Job drawing, mm, ordinate dimensions from the low corner. One solid piece. Give positions to 0.01 mm unless a question says otherwise; leave off trailing zeros. Order: outer loops, then holes, each group sorted by start corner. A loop starts at its lowest first (then second) coordinate and runs counter-clockwise, first axis right, second up. Notation, with made-up numbers: (28.25, 14) -> (77.25, 14) arc R22 ccw to (77.25, 42) -> close; hole circle Ø4 at (47, 51). An arc over 180 degrees is marked (long way). Write item = value, one per line. Start each with the question number.
(1) Two-plate mould, pull along X, no slides. Class the marked faces 1, 2 and 3: pulls with the +X half, pulls with the -X half, needs draft (parallel to the pull), parting line crosses it, or undercut.
(2) Saw through at A-A, the plane y = 12.5. List the corners of the cut face in (x, z).
(3) Saw through at C-C, the plane x = 8.25. State how many separate pieces and enclosed holes the cut face has, then the cut area to 3 significant figures.
(4) Probe line 1 along Y through (x, z) = (11.5, 14.5); line 2 along Y through (x, z) = (18.75, 17) (1 decimal); line 3 along X through (y, z) = (8, 10.25). List the from-to ranges inside material, lowest first. Write a range as from..to.
(5) Flat gauge pin, fed straight in: pin 1 (2.5 mm diameter, centred on y = 2.46, z = 2.7, fed in from -X). Where does the tip first touch, or does it go through?
(6) Saw through at B-B, the plane z = 7.75. List the corners of the cut face in (x, y), then the cut area to 3 significant figures.
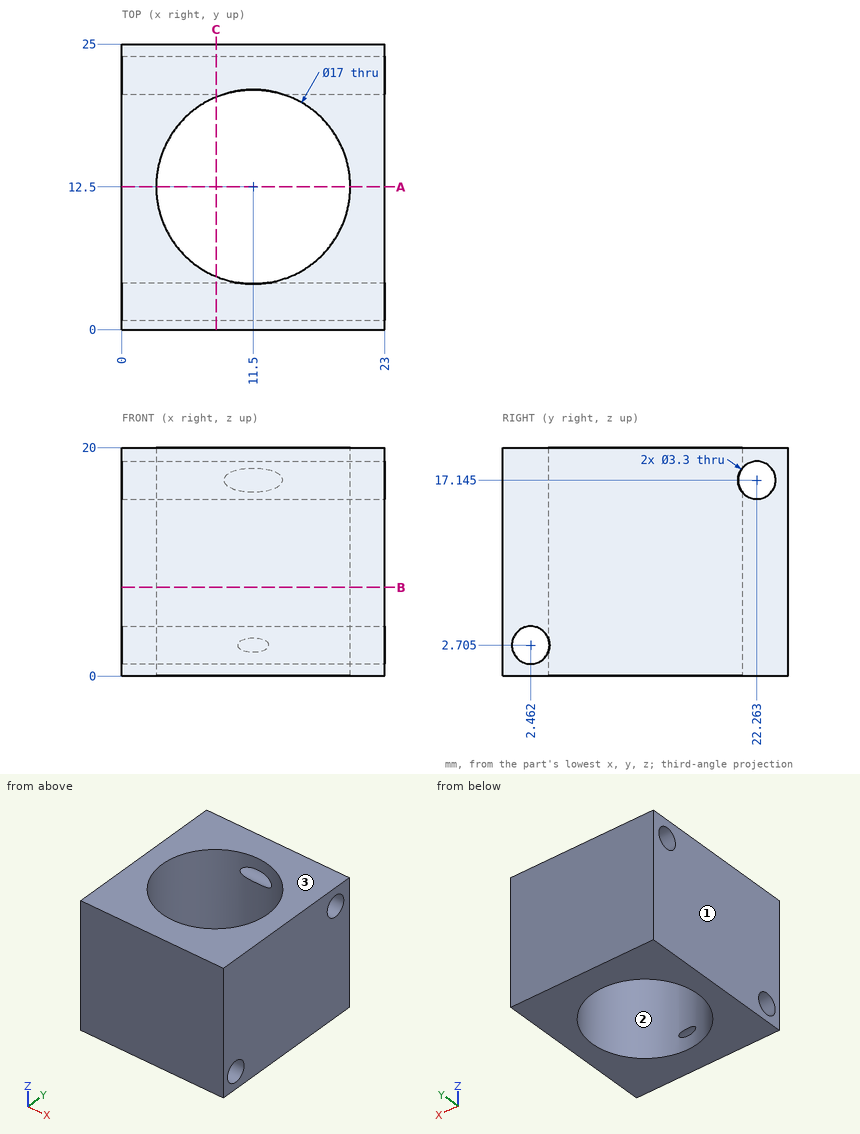
Results list:
q1.face_1 = pulls with the -X half
q1.face_2 = undercut
q1.face_3 = needs draft
q2.outline = (0, 0) -> (3, 0) -> (3, 20) -> (0, 20) -> close; (20, 0) -> (23, 0) -> (23, 20) -> (20, 20) -> close
q3.separate_pieces = 2
q3.enclosed_holes = 2
q3.area = 169 mm^2
q4.line_1 = 0..4, 21..25
q4.line_2 = 0..8.1, 16.9..20.6, 23.9..25
q4.line_3 = 0..4.29, 18.71..23
q5.pin_1 = through
q6.outline = (0, 0) -> (23, 0) -> (23, 25) -> (0, 25) -> close; hole circle Ø17 at (11.5, 12.5)
q6.area = 348 mm^2
